Design review of the part built by this model. Coordinates are the model's own, in mm. Face numbers are marked on the shaded views. A direction names the side the tool comes from. Give positions to 0.01 mm unless a question says otherwise; leave off trailing zeros. Write each loop counter-clockwise with the first axis right and the second up, starting at its lowest first coordinate (ties: lowest second). Pieces come first, ordered by that corner, then holes.
```python
from build123d import *

# Parameters (mm, degrees)
EXTRUDE_1_DEPTH     = 6
CUT_EXTRUDE_1_DEPTH = 4
SKETCH_3_R          = 1.5
CUT_EXTRUDE_2_DEPTH = 20
EXTRUDE_2_DEPTH     = 10
EXTRUDE_3_DEPTH     = 10
SKETCH_5_W          = 3
SKETCH_5_H          = 6
CUT_EXTRUDE_3_DEPTH = 52.778373864


with BuildPart() as part:
    # Эскиз1 → Бобышка-Вытянуть1 (new body)
    with BuildSketch(Plane.XY):
        with BuildLine():
            Line((0, 10), (0, 5))
            ThreePointArc((0, 5), (3.535533906, 3.535533906), (5, 0))
            ThreePointArc((5, 0), (3.535533906, -3.535533906), (0, -5))
            Line((0, -5), (0, -10))
            ThreePointArc((0, -10), (7.071067812, -7.071067812), (10, 0))
            ThreePointArc((10, 0), (7.071067812, 7.071067812), (0, 10))
        make_face()
        with BuildLine():
            ThreePointArc((0, -5), (-3.535533906, -3.535533906), (-5, 0))
            Line((-5, 0), (-10, 0))
            ThreePointArc((-10, 0), (-7.071067812, -7.071067812), (0, -10))
            Line((0, -10), (0, -5))
        make_face()
        with BuildLine():
            Line((-10, 0), (-5, 0))
            ThreePointArc((-5, 0), (-3.535533906, 3.535533906), (0, 5))
            Line((0, 5), (0, 10))
            ThreePointArc((0, 10), (-7.071067812, 7.071067812), (-10, 0))
        make_face()
        with BuildLine():
            ThreePointArc((0, -10), (-7.071067812, -7.071067812), (-10, 0))
            Line((-10, 0), (-50, 0))
            Line((-50, 0), (-50, -10))
            Line((-50, -10), (0, -10))
        make_face()
        with BuildLine():
            Line((-50, 0), (-10, 0))
            ThreePointArc((-10, 0), (-7.071067812, 7.071067812), (0, 10))
            Line((0, 10), (-50, 10))
            Line((-50, 10), (-50, 0))
        make_face()
    extrude(amount=EXTRUDE_1_DEPTH)

    # Эскиз2 → Вырез-Вытянуть1 (cut)
    with BuildSketch(Plane.XY.offset(6)):
        with BuildLine():
            Line((-4.385462329, 4.661300265), (-17.4, 2.6))
            ThreePointArc((-17.4, 2.6), (-20, 0), (-17.4, -2.6))
            Line((-17.4, -2.6), (-4.385462329, -4.661300265))
            ThreePointArc((-4.385462329, -4.661300265), (6.4, 0), (-4.385462329, 4.661300265))
        make_face()
    extrude(amount=-CUT_EXTRUDE_1_DEPTH, mode=Mode.SUBTRACT)

    # Эскиз3 → Вырез-Вытянуть2 (cut)
    with BuildSketch(Plane.ZY.offset(50)):
        with Locations((2.2, 5)):
            Circle(SKETCH_3_R)
        with Locations((2.2, -5)):
            Circle(SKETCH_3_R)
    extrude(amount=-CUT_EXTRUDE_2_DEPTH, mode=Mode.SUBTRACT)

    # Эскиз4 → Бобышка-Вытянуть2 (add, symmetric)
    with BuildSketch(Plane(origin=(0, 0, 0), x_dir=(1, 0, 0), z_dir=(0, 1, 0))):
        Polygon((-50, 0), (-24, 0), (-26, 2), (-50, 2), align=None)
    extrude(amount=EXTRUDE_2_DEPTH, both=True)

    # Эскиз6 → Бобышка-Вытянуть3 (add, symmetric)
    with BuildSketch(Plane(origin=(0, 0, 0), x_dir=(1, 0, 0), z_dir=(0, 1, 0))):
        Polygon((-24, -6), (-50, -6), (-50, -7), (-25, -7), align=None)
    extrude(amount=EXTRUDE_3_DEPTH, both=True)

    # Эскиз5 → Вырез-Вытянуть3 (cut, through all)
    with BuildSketch(Plane(origin=(0, 0, -2), x_dir=(-1, 0, 0), z_dir=(0, 0, -1))):
        with Locations((36.5, -5)):
            Rectangle(SKETCH_5_W, SKETCH_5_H)
        with Locations((36.5, 5)):
            Rectangle(SKETCH_5_W, SKETCH_5_H)
    extrude(amount=-CUT_EXTRUDE_3_DEPTH, mode=Mode.SUBTRACT)


solid = part.part
```
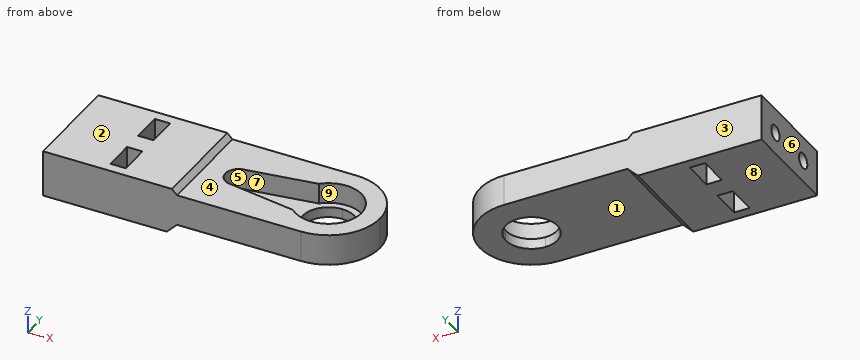
(1) Clearance check with flat-ended pins moving along their axes: P1, Ø3.5, axis at y = 5, z = 2.2, coming from the +X side; P2, Ø1.8, axis at y = -5, z = 2, coming from the +X side; P3, Ø2, axis at x = -3, y = -6.5, coming from the -Z side. State where each tip first meets the part, or that it passes through.
Resolved:
P1: stops at x = 9.46
P2: stops at x = 9.12
P3: stops at z = 0
(2) Consider section A-A, the plane x = -39. Give the boundary of the cut face in (y, z).
Resolved:
outline: (-10, -2) - (10, -2) - (10, 7) - (-10, 7) - close; hole circle Ø3 at (-5, 2.2); hole circle Ø3 at (5, 2.2)
(3) Mouldability with a two-part tool opening along X and no side actions: class the marked faces 6, 7, 8 and 9 as pulls with the +X half, pulls with the -X half, needs draft (parallel to the pull), parting line crosses it, or undercut.
Resolved:
face 6: pulls with the -X half
face 7: undercut
face 8: needs draft
face 9: undercut
(4) Tool access review of the marked faces 1, 2, 3, 4 and 5: name each direction out of +Z, -Z, +X, -X, +Y, -Y from which nothing blocks a thin tool from reaching the whole face with its end or side.
Resolved:
face 1: -Z, +X, +Y, -Y
face 2: +Z, +X, -X, +Y, -Y
face 3: +Z, -Z, +X, -X, +Y
face 4: +Z, +X, +Y, -Y
face 5: +Z
(5) To check wall thickness, follow L1, parallel to Y at x = -33.85, z = 2.2; L2, parallel to Y at x = -35.5, z = 6.25; L3, parallel to X at y = 3.25, z = 1.25. State the ranges of each line that lie inside material, in increasing order.
Resolved:
L1: y = -10 to -6.5, -3.5 to 3.5, 6.5 to 10
L2: y = -10 to -8, -2 to 2, 8 to 10
L3: x = -50 to -38, -35 to -3.8, 3.8 to 9.46
(6) Consider section C-C, the plane x = -16.5. Give the boundary of the cut face in (y, z), then the cut area to 3 significant figures.
Resolved:
outline: (-10, 0) - (10, 0) - (10, 6) - (2.74, 6) - (2.74, 2) - (-2.74, 2) - (-2.74, 6) - (-10, 6) - close
area: 98.1 mm2
